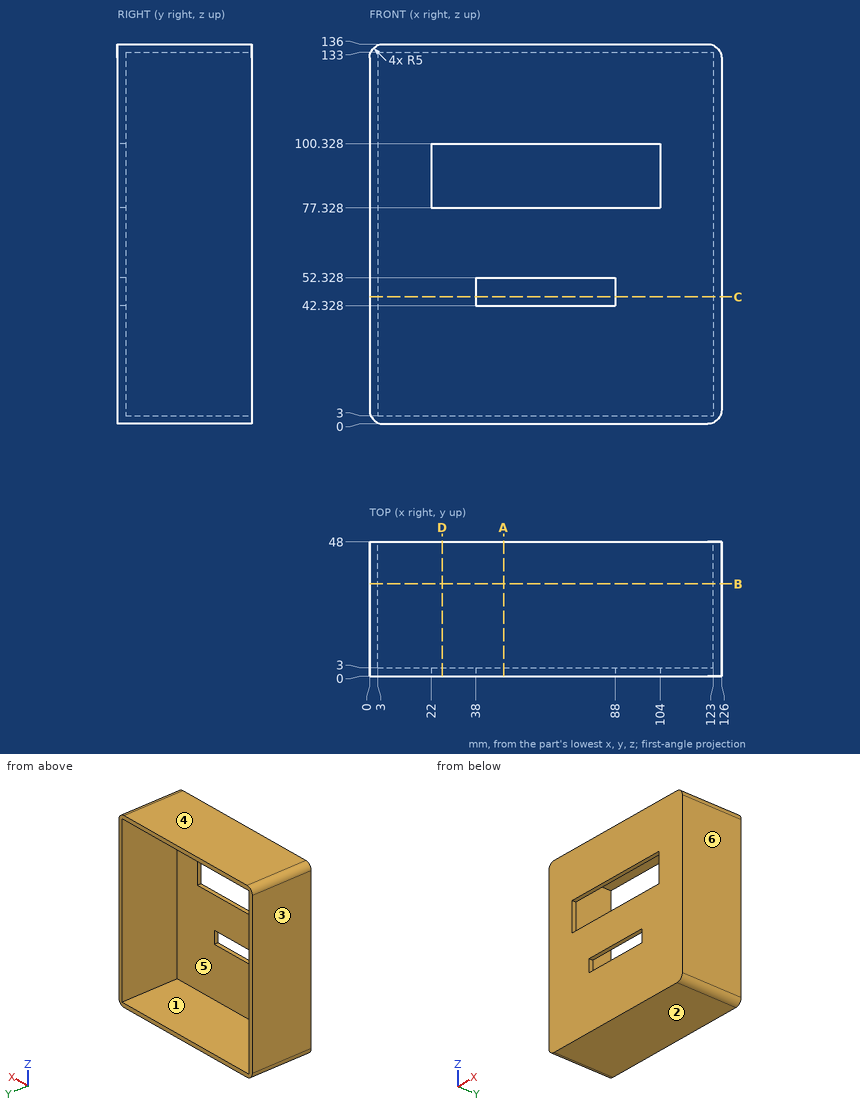
Input: dimensioned drawing with shaded views. Units: mm. Origin: part minimum x, y, z. A direction names the side the tool comes from. Coordinates: 2 decimals unless noted, no trailing zeros. Loops run counter-clockwise (first coordinate to the right, second up) from the corner with the lowest first, then second, coordinate; pieces in that order, holes last. Notation, with made-up numbers: (9.25, -31.5) -> (16.25, -31.5) arc R15 ccw to (16.25, -3.5) -> close; hole circle Ø2 at (62.25, 14). An arc over 180 degrees is marked (long way). One line per item, written item: value. Start each with the question number.
Q1. Section query A-A, the plane x = 48. Return the cut outline in (y, z), and give its area (3 significant figures).
Q2. Section query B-B, the plane y = 33. Return the cut outline in (x, z).
Q3. Section query C-C, the plane z = 45.5. Return the cut outline in (x, y), and give its area (3 significant figures).
Q4. Contact query for a flat-ended pin moving along its axis: P1, Ø12, axis at x = 38, z = 82, coming from the +Y side. Output: stop coordinate, or through.
Q5. Line query: line 1 along Z through (x, y) = (50, 28.5); line 2 along X through (y, z) = (19.5, 33.5); line 3 along Y through (x, z) = (111, 119). Output: solid intervals per line, ascending.
Q6. Set-up query: the marked faces 1 and 2. Return all of +Z, -Z, +X, -X, +Y, -Y with unobstructed straight access to the full face (end or side cutting, diameter ignored); none if empty.
Q7. Section query D-D, the plane x = 26. Return the cut outline in (y, z).
Q8. Mould query, pull axis X, two halves, no side actions, for the marked faces 3, 4, 5 and 6. Classes: pulls with the +X half, pulls with the -X half, needs draft (parallel to the pull), parting line crosses it, or undercut.
Results:
1. outline: (0, 0) -> (48, 0) -> (48, 3) -> (3, 3) -> (3, 42.33) -> (0, 42.33) -> close; (0, 52.33) -> (3, 52.33) -> (3, 77.33) -> (0, 77.33) -> close; (0, 100.33) -> (3, 100.33) -> (3, 133) -> (48, 133) -> (48, 136) -> (0, 136) -> close
1. area: 579 mm^2
2. outline: (0, 5) arc R5 ccw to (5, 0) -> (121, 0) arc R5 ccw to (126, 5) -> (126, 131) arc R5 ccw to (121, 136) -> (5, 136) arc R5 ccw to (0, 131) -> close; hole (3, 3) -> (123, 3) -> (123, 133) -> (3, 133) -> close
3. outline: (0, 0) -> (38, 0) -> (38, 3) -> (3, 3) -> (3, 48) -> (0, 48) -> close; (88, 0) -> (126, 0) -> (126, 48) -> (123, 48) -> (123, 3) -> (88, 3) -> close
3. area: 498 mm^2
4. P1: y = 3
5. line 1: 0 to 3, 133 to 136
5. line 2: 0 to 3, 123 to 126
5. line 3: 0 to 3
6. face 1: +Y
6. face 2: -Z, +X, -X, +Y, -Y
7. outline: (0, 0) -> (48, 0) -> (48, 3) -> (3, 3) -> (3, 77.33) -> (0, 77.33) -> close; (0, 100.33) -> (3, 100.33) -> (3, 133) -> (48, 133) -> (48, 136) -> (0, 136) -> close
8. face 3: pulls with the -X half
8. face 4: needs draft
8. face 5: undercut
8. face 6: pulls with the +X half
